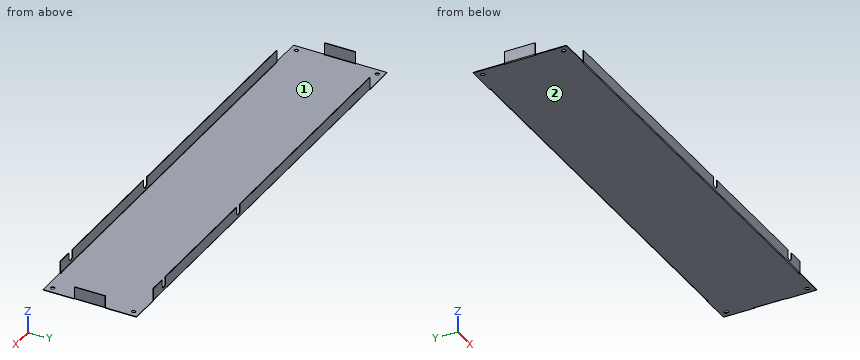
```python
from build123d import *

# Parameters (mm, degrees)
SKETCH_1_W                        = 730
SKETCH_1_H                        = 149
SKETCH_1_R                        = 3
SM_BASE_FLANGE_1_DEPTH            = 0.8
SM_EDGE_FLANGE_1_STRIP_W          = 4.2
SM_EDGE_FLANGE_1_STRIP_H          = 0.8
SM_EDGE_FLANGE_1_STRIP_CUT_DEPTH  = 49
SM_EDGE_FLANGE_1_RELIEF_W         = 5
SM_EDGE_FLANGE_1_RELIEF_H         = 0.8
SM_EDGE_FLANGE_1_RELIEF_CUT_DEPTH = 0.8
SM_EDGE_FLANGE_1_DEPTH            = 49
SM_EDGE_FLANGE_2_STRIP_W          = 4.2
SM_EDGE_FLANGE_2_STRIP_H          = 0.8
SM_EDGE_FLANGE_2_STRIP_CUT_DEPTH  = 49
SM_EDGE_FLANGE_2_RELIEF_W         = 5
SM_EDGE_FLANGE_2_RELIEF_H         = 0.8
SM_EDGE_FLANGE_2_RELIEF_CUT_DEPTH = 0.8
SM_EDGE_FLANGE_2_DEPTH            = 49
SM_EDGE_FLANGE_3_STRIP_W          = 4.2
SM_EDGE_FLANGE_3_STRIP_H          = 0.8
SM_EDGE_FLANGE_3_STRIP_CUT_DEPTH  = 630
SM_EDGE_FLANGE_3_RELIEF_W         = 5
SM_EDGE_FLANGE_3_RELIEF_H         = 0.8
SM_EDGE_FLANGE_3_RELIEF_CUT_DEPTH = 0.8
SM_EDGE_FLANGE_3_DEPTH            = 630
SM_EDGE_FLANGE_3_FLAT_DEPTH       = 0.8


# Sheet-metal steps are written as plain solids
with BuildPart() as part:
    # Sketch 1 → 基体-法兰1 (new body)
    with BuildSketch(Plane.XY):
        Rectangle(SKETCH_1_W, SKETCH_1_H)
        with Locations((-355, 64.5)):
            Circle(SKETCH_1_R, mode=Mode.SUBTRACT)
        with Locations((-355, -64.5)):
            Circle(SKETCH_1_R, mode=Mode.SUBTRACT)
        with Locations((355, 64.5)):
            Circle(SKETCH_1_R, mode=Mode.SUBTRACT)
        with Locations((355, -64.5)):
            Circle(SKETCH_1_R, mode=Mode.SUBTRACT)
    extrude(amount=-SM_BASE_FLANGE_1_DEPTH)

    # 边线-法兰1 strip (across the edge) → 边线-法兰1 strip cut (cut)
    with BuildSketch(Plane(origin=(-365, 24.5, 0), x_dir=(1, 0, 0), z_dir=(0, -1, 0))):
        with Locations((-0.8, -0.4)):
            Rectangle(SM_EDGE_FLANGE_1_STRIP_W, SM_EDGE_FLANGE_1_STRIP_H)
    extrude(amount=SM_EDGE_FLANGE_1_STRIP_CUT_DEPTH, mode=Mode.SUBTRACT)

    # 边线-法兰1 relief (on the sheet) → 边线-法兰1 relief cut (cut)
    with BuildSketch(Plane(origin=(-363.7, 24.5, 0), x_dir=(1, 0, 0), z_dir=(0, 0, 1))):
        with Locations((-1.7, 0.4)):
            Rectangle(SM_EDGE_FLANGE_1_RELIEF_W, SM_EDGE_FLANGE_1_RELIEF_H)
        with Locations((-1.7, -49.4)):
            Rectangle(SM_EDGE_FLANGE_1_RELIEF_W, SM_EDGE_FLANGE_1_RELIEF_H)
    extrude(amount=-SM_EDGE_FLANGE_1_RELIEF_CUT_DEPTH, mode=Mode.SUBTRACT)

    # 边线-法兰1 section (across the edge) → 边线-法兰1 (add)
    with BuildSketch(Plane(origin=(-365, 24.5, 0), x_dir=(1, 0, 0), z_dir=(0, -1, 0))):
        with BuildLine():
            Line((0, 0.5), (0, 19.2))
            Line((0, 19.2), (0.8, 19.2))
            Line((0.8, 19.2), (0.8, 0.5))
            ThreePointArc((0.8, 0.5), (0.946446609, 0.146446609), (1.3, 0))
            Line((1.3, 0), (1.3, -0.8))
            ThreePointArc((1.3, -0.8), (0.380761184, -0.419238816), (0, 0.5))
        make_face()
    extrude(amount=SM_EDGE_FLANGE_1_DEPTH)

    # 边线-法兰2 strip (across the edge) → 边线-法兰2 strip cut (cut)
    with BuildSketch(Plane(origin=(365, -24.5, 0), x_dir=(-1, 0, 0), z_dir=(0, 1, 0))):
        with Locations((-0.8, -0.4)):
            Rectangle(SM_EDGE_FLANGE_2_STRIP_W, SM_EDGE_FLANGE_2_STRIP_H)
    extrude(amount=SM_EDGE_FLANGE_2_STRIP_CUT_DEPTH, mode=Mode.SUBTRACT)

    # 边线-法兰2 relief (on the sheet) → 边线-法兰2 relief cut (cut)
    with BuildSketch(Plane(origin=(363.7, -24.5, 0), x_dir=(-1, 0, 0), z_dir=(0, 0, 1))):
        with Locations((-1.7, 0.4)):
            Rectangle(SM_EDGE_FLANGE_2_RELIEF_W, SM_EDGE_FLANGE_2_RELIEF_H)
        with Locations((-1.7, -49.4)):
            Rectangle(SM_EDGE_FLANGE_2_RELIEF_W, SM_EDGE_FLANGE_2_RELIEF_H)
    extrude(amount=-SM_EDGE_FLANGE_2_RELIEF_CUT_DEPTH, mode=Mode.SUBTRACT)

    # 边线-法兰2 section (across the edge) → 边线-法兰2 (add)
    with BuildSketch(Plane(origin=(365, -24.5, 0), x_dir=(-1, 0, 0), z_dir=(0, 1, 0))):
        with BuildLine():
            Line((0, 0.5), (0, 19.2))
            Line((0, 19.2), (0.8, 19.2))
            Line((0.8, 19.2), (0.8, 0.5))
            ThreePointArc((0.8, 0.5), (0.946446609, 0.146446609), (1.3, 0))
            Line((1.3, 0), (1.3, -0.8))
            ThreePointArc((1.3, -0.8), (0.380761184, -0.419238816), (0, 0.5))
        make_face()
    extrude(amount=SM_EDGE_FLANGE_2_DEPTH)

    # 边线-法兰3 strip (across the edge) → 边线-法兰3 strip cut (cut)
    with BuildSketch(Plane(origin=(315, 74.5, 0), x_dir=(0, -1, 0), z_dir=(-1, 0, 0))):
        with Locations((-0.8, -0.4)):
            Rectangle(SM_EDGE_FLANGE_3_STRIP_W, SM_EDGE_FLANGE_3_STRIP_H)
    sm_edge_flange_3_strip_cut = extrude(amount=SM_EDGE_FLANGE_3_STRIP_CUT_DEPTH, mode=Mode.SUBTRACT)

    # 边线-法兰3 relief (on the sheet) → 边线-法兰3 relief cut (cut)
    with BuildSketch(Plane(origin=(315, 73.2, 0), x_dir=(0, -1, 0), z_dir=(0, 0, 1))):
        with Locations((-1.7, 0.4)):
            Rectangle(SM_EDGE_FLANGE_3_RELIEF_W, SM_EDGE_FLANGE_3_RELIEF_H)
        with Locations((-1.7, -630.4)):
            Rectangle(SM_EDGE_FLANGE_3_RELIEF_W, SM_EDGE_FLANGE_3_RELIEF_H)
    sm_edge_flange_3_relief_cut = extrude(amount=-SM_EDGE_FLANGE_3_RELIEF_CUT_DEPTH, mode=Mode.SUBTRACT)

    # 边线-法兰3 bend section (across the edge) → 边线-法兰3 (add)
    with BuildSketch(Plane(origin=(315, 74.5, 0), x_dir=(0, -1, 0), z_dir=(-1, 0, 0))):
        with BuildLine():
            Line((0, 0.5), (0.8, 0.5))
            ThreePointArc((0.8, 0.5), (0.946446609, 0.146446609), (1.3, 0))
            Line((1.3, 0), (1.3, -0.8))
            ThreePointArc((1.3, -0.8), (0.380761184, -0.419238816), (0, 0.5))
        make_face()
    sm_edge_flange_3 = extrude(amount=SM_EDGE_FLANGE_3_DEPTH)

    # 边线-法兰3 profile (on flange) → 边线-法兰3 flat (add)
    with BuildSketch(Plane(origin=(0, 74.5, 0), x_dir=(-1, 0, 0), z_dir=(0, 1, 0))):
        with BuildLine():
            Line((-315, 0.5), (315, 0.5))
            Line((315, 0.5), (315, 19.2))
            Line((315, 19.2), (-63, 19.2))
            Line((-63, 19.2), (-63, 9.2))
            ThreePointArc((-63, 9.2), (-68, 4.2), (-73, 9.2))
            Line((-73, 9.2), (-73, 19.2))
            Line((-73, 19.2), (-280, 19.2))
            Line((-280, 19.2), (-280, 9.2))
            ThreePointArc((-280, 9.2), (-285, 4.2), (-290, 9.2))
            Line((-290, 9.2), (-290, 19.2))
            Line((-290, 19.2), (-315, 19.2))
            Line((-315, 19.2), (-315, 0.5))
        make_face()
    sm_edge_flange_3_flat = extrude(amount=-SM_EDGE_FLANGE_3_FLAT_DEPTH)

    # 镜向1: 边线-法兰3 strip cut, 边线-法兰3 relief cut, 边线-法兰3, 边线-法兰3 flat across plane
    add(sm_edge_flange_3_strip_cut.mirror(Plane.ZX), mode=Mode.SUBTRACT)
    add(sm_edge_flange_3_relief_cut.mirror(Plane.ZX), mode=Mode.SUBTRACT)
    add(sm_edge_flange_3.mirror(Plane.ZX))
    add(sm_edge_flange_3_flat.mirror(Plane.ZX))


solid = part.part
```
Check sheet for the modelled part. Datum: model origin and axes. Units: mm. Face numbers are marked on the shaded views. A direction names the side the tool comes from. Coordinates: 2 decimals unless noted, no trailing zeros. Order: outer loops, then holes, each group sorted by start corner. A loop starts at its lowest first (then second) coordinate and runs counter-clockwise, first axis right, second up. Notation, with made-up numbers: M 49.5,26 L 93.5,26 A9 ccw 93.5,39 Z; hole C 39,-11 d5. An arc over 180 degrees is marked long. One line per question, with ' | ' between items. Start each with the question number.
Item 1: Sectioned sample at C-C on y = -35. Record the cut outline in (x, z).
Item 2: Sectioned sample at A-A on z = 12.25. Count the separate pieces of the cut face and the enclosed holes in it, and give its area (3 significant figures).
Item 3: Gauge pin test, flat ends, axial feed: P1, Ø0.6, axis at x = 364, z = 14, coming from the -Y side; P2, Ø0.9, axis at y = -25, z = -0.5, coming from the -X side; P3, Ø1.7, axis at y = 73, z = 5.5, coming from the -X side; P4, Ø2.5, axis at y = 73, z = 9.5, coming from the +X side. Record the tip position at first contact, or that the pin passes through.
Item 4: Access from +Z, -Z, +X, -X, +Y, -Y to the whole of each face (thin tool, end or side, straight path). Record for the marked faces 1 and 2.
Item 5: Sectioned sample at B-B on x = 53. Record the cut outline in (y, z), and give its area (3 significant figures).
Item 6: Material ranges on line 1 (Y direction, x = -355, z = -0.55); line 2 (Y direction, x = -257, z = 6.25); line 3 (X direction, y = 22.5, z = 0.5), recorded low to high.
Answer below:
1) outline: M -365,-0.8 L 365,-0.8 L 365,0 L -365,0 Z
2) separate pieces: 8 | enclosed holes: 0 | area: 1,050 mm^2
3) P1: stops at y = -24.5 | P2: stops at x = -365 | P3: stops at x = -315 | P4: stops at x = 315
4) face 1: +Z | face 2: -Z, +X, -X, +Y, -Y
5) outline: M -74.5,0.5 A1.3 ccw -73.2,-0.8 L 73.2,-0.8 A1.3 ccw 74.5,0.5 L 74.5,19.2 L 73.7,19.2 L 73.7,0.5 A0.5 cw 73.2,0 L -73.2,0 A0.5 cw -73.7,0.5 L -73.7,19.2 L -74.5,19.2 Z | area: 149 mm^2
6) line 1: y = -74.5 to -67.5, -61.5 to 61.5, 67.5 to 74.5 | line 2: y = -74.5 to -73.7, 73.7 to 74.5 | line 3: x = -365 to -364.2, 364.2 to 365
